Check sheet for the modelled part. Datum: model origin and axes. Units: mm. A direction names the side the tool comes from. Give positions to 0.01 mm unless a question says otherwise; leave off trailing zeros. Order: outer loops, then holes, each group sorted by start corner. A loop starts at its lowest first (then second) coordinate and runs counter-clockwise, first axis right, second up. Notation, with made-up numbers: M 63.25,16 L 100.25,16 A16 cw 100.25,24 Z; hole C 72,60.5 d7. An arc over 180 degrees is marked long. Return JSON: item names as keys, results as strings. Group by question number.
from build123d import *

# Parameters (mm, degrees)
P_IDAT_VYSUNUT_M1_DEPTH  = 3
P_IDAT_VYSUNUT_M2_DEPTH  = 2
ZAOBLIT4_R               = 1
SKICA2_W                 = 4
SKICA2_H                 = 2
ODEBRAT_VYSUNUT_M2_DEPTH = 0.8
SKICA3_W                 = 4
SKICA3_H                 = 2
ODEBRAT_VYSUNUT_M3_DEPTH = 0.8


with BuildPart() as part:
    # Skica1 → P_idat vysunut_m1 (new body)
    with BuildSketch(Plane(origin=(0, 0, 0), x_dir=(1, 0, 0), z_dir=(0, 1, 0))):
        Polygon((-118.143750166, 15), (-118.143750166, 0), (-68.779346971, 32.313398106), (-16.32734533, 12.51119421), (-26.593132493, 30.830954414), (-20.343228113, 42.230019956), (0, 37.22), (0, 69.22), (-39.317553332, 46.52), (-78.635106664, 69.22), (-118.143185584, 46.41), (-118.143185584, 33.5570142), (-107.643750166, 37.378496169), (-107.643750166, 24.278496169), (-128.093750166, 24.278496169), (-128.093750166, 11.378496169), align=None)
    extrude(amount=P_IDAT_VYSUNUT_M1_DEPTH)

    # Skica1_5 → P_idat vysunut_m2 (add)
    with BuildSketch(Plane(origin=(0, 0, 0), x_dir=(1, 0, 0), z_dir=(0, 1, 0))):
        Polygon((-68.779346971, 32.313398106), (-118.143750166, 0), (0, 0), (0, 15), (9.950504516, 11.37831254), (9.950504516, 24.27831254), (-10.5, 24.27831254), (-10.5, 37.37831254), (0, 33.55662508), (0, 37.22), (-20.343228113, 42.230019956), (-26.593132493, 30.830954414), (-16.32734533, 12.51119421), align=None)
    extrude(amount=P_IDAT_VYSUNUT_M2_DEPTH)

    # Zaoblit4
    zaoblit4_edges = [part.edges().sort_by_distance(p)[0] for p in [
        (-118.143750166, 1.5, -15),
        (-128.093750166, 1.5, -11.378496169),
        (-128.093750166, 1.5, -24.278496169),
        (-107.643750166, 1.5, -24.278496169),
        (-107.643750166, 1.5, -37.378496169),
        (-118.143185584, 1.5, -33.5570142),
        (-10.5, 1, -24.27831254),
        (-10.5, 1, -37.37831254),
        (0, 1, -33.55662508),
        (0, 1, -15),
        (9.950504516, 1, -11.37831254),
        (9.950504516, 1, -24.27831254),
    ]]
    fillet(zaoblit4_edges, radius=ZAOBLIT4_R)

    # Skica2 → Odebrat vysunut_m2 (cut)
    with BuildSketch(Plane(origin=(0, 3, 0), x_dir=(1, 0, 0), z_dir=(0, 1, 0))):
        with Locations((-126.093750166, 15.742570172)):
            Rectangle(SKICA2_W, SKICA2_H)
        Polygon((-103.64375629, 27.314422166), (-107.643750166, 27.321421806), (-107.643750166, 29.314422166), (-103.643750166, 29.314422166), align=None)
        Polygon((-103.64375629, 33.914422166), (-107.643750166, 33.907422526), (-107.643750166, 31.914422166), (-103.643750166, 31.914422166), align=None)
    extrude(amount=-ODEBRAT_VYSUNUT_M2_DEPTH, mode=Mode.SUBTRACT)

    # Skica3 → Odebrat vysunut_m3 (cut)
    with BuildSketch(Plane(origin=(0, 2, 0), x_dir=(1, 0, 0), z_dir=(0, 1, 0))):
        with Locations((7.950504516, 15.742386544)):
            Rectangle(SKICA3_W, SKICA3_H)
        with Locations((7.950504516, 20.342386544)):
            Rectangle(SKICA3_W, SKICA3_H)
    extrude(amount=-ODEBRAT_VYSUNUT_M3_DEPTH, mode=Mode.SUBTRACT)


solid = part.part
1) Tool access check on faces 4 (the face through (-118.143, 1, -41)), 5 (the face through (-42.92, 2.49, -22.55)), 6 (the face through (4.92, 0.99, -13.21)), 7 (the face through (-23.512, 2.493, -36.451)), 8 (the face through (-19.38, 1.48, -58.03)). Record the directions out of +Z, -Z, +X, -X, +Y, -Y that give a thin tool (end or side, any length) a straight path to the whole face; none if there is none.
2) Depth check by flat-ended pin: P1, Ø0.6, axis at x = -105, z = -28, coming from the +Y side; P2, Ø0.9, axis at x = -105, y = 2.5, coming from the -Z side; P3, Ø1, axis at x = -1, y = 1, coming from the -Z side; P4, Ø3, axis at x = -28.5, z = -41, coming from the -Y side. Enter the tip coordinate at first touch or a pass-through.
3) Material ranges on line 1 along Z through (x, y) = (-104, 2.65); line 2 along X through (y, z) = (1.8, -19.5); line 3 along X through (y, z) = (1.85, -11.5), recorded low to high.
4) Sectioned sample at B-B on x = -3.5. Record the boundary of the cut face in (y, z), then the cut area to 3 significant figures.
5) Sectioned sample at D-D on z = -44.5. Record the boundary of the cut face in (x, y).
6) Release check for a two-part mould opening along X. For faces 1 (the face through (-118, 1, -24.278)), 2 (the face through (-107.644, 1, -31)), 3 (the face through (-21.388, 2.493, -21.543)) record: released by +X, released by -X, zero draft, split by the parting line, or undercut.
7) Sectioned sample at A-A on z = -55.5. Record the boundary of the cut face in (x, y), then the cut area to 3 significant figures.
Reply:
{
 "1": {"face 4": "-Z, -X, +Y, -Y", "face 5": "+Z, +Y", "face 6": "+Z, +Y, -Y", "face 7": "+Y", "face 8": "-Z, +Y, -Y"},
 "2": {"P1": "y = 2.2", "P2": "z = -54.26", "P3": "z = -68.93", "P4": "y = 0"},
 "3": {"line 1": "-54.58 to -33.91, -31.91 to -29.31, -27.32 to -9.26", "line 2": "-128.09 to 5.95", "line 3": "-118.14 to 0"},
 "4": {"outline": "M 0,-67.2 L 3,-67.2 L 3,-38.08 L 2,-38.08 L 2,-34.83 L 0,-34.83 Z; M 0,-24.28 L 2,-24.28 L 2,0 L 0,0 Z", "area": "142 mm^2"},
 "5": {"outline": "M -118.14,0 L 0,0 L 0,3 L -118.14,3 Z"},
 "6": {"face 1": "zero draft", "face 2": "undercut", "face 3": "released by +X"},
 "7": {"outline": "M -102.4,0 L -54.87,0 L -54.87,3 L -102.4,3 Z; M -23.76,0 L 0,0 L 0,3 L -23.76,3 Z", "area": "214 mm^2"}
}
